Build history of the part. All positions in model axes, mm. Round coordinates to 2 decimals unless told otherwise and drop trailing zeros. Write each question's results on one line, items separated by ' | '. Start each with the question number.
```python
from build123d import *

# Parameters (mm, degrees)
SKETCH1_W            = 203.2
SKETCH1_H            = 177.8
SKETCH1_W_2          = 15.24
SKETCH1_H_2          = 17.78
BOSS_EXTRUDE1_DEPTH  = 2.54
LPATTERN2_COUNT      = 9
LPATTERN2_PITCH      = 20
LPATTERN2_COUNT_DIR2 = 10
LPATTERN2_PITCH_DIR2 = 20


with BuildPart() as part:
    # Sketch1 → Boss-Extrude1 (new body)
    with BuildSketch(Plane.XY):
        Rectangle(SKETCH1_W, SKETCH1_H)
        with Locations((-30.48, 0)):
            Rectangle(SKETCH1_W_2, SKETCH1_H_2, mode=Mode.SUBTRACT)
        with Locations((30.48, 0)):
            Rectangle(SKETCH1_W_2, SKETCH1_H_2, mode=Mode.SUBTRACT)
    extrude(amount=BOSS_EXTRUDE1_DEPTH)

    # Sketch4 → M2.5 Clearance Hole1 (revolve, cut)
    with BuildSketch(Plane(origin=(91.6, 78.994, 0), x_dir=(0, 1, 0), z_dir=(1, 0, 0))):
        Polygon((0, 0), (0, 5.623506083), (1.75, 4.572), (1.75, 0), align=None)
    m2_5_clearance_hole1 = revolve(axis=Axis((91.6, 78.994, -6.35), (0, 0, 1)), mode=Mode.SUBTRACT)

    # LPattern2: M2.5 Clearance Hole1 9 × 10, 8 skipped
    with Locations(*[(-j * LPATTERN2_PITCH_DIR2, -i * LPATTERN2_PITCH, 0) for i in range(LPATTERN2_COUNT) for j in range(LPATTERN2_COUNT_DIR2) if (i, j) not in ((0, 0), (4, 3), (4, 4), (4, 5), (4, 6), (5, 3), (5, 4), (5, 5), (5, 6))]):
        add(m2_5_clearance_hole1, mode=Mode.SUBTRACT)


solid = part.part
```
Item 1: Saw through at A-A, the plane z = 1.4. State how many separate pieces and enclosed holes the cut face has, then the cut area to 3 significant figures.
Item 2: Drill centre line: line 1 along X through (y, z) = (-6.5, 1.55). Where is it in solid material? Low to high. Write a range as [from, to].
Item 3: Drop a flat-ended pin along its axis: pin 1 (3 mm diameter, centred on x = 51.6, y = -21.006, fed in from -Z). Give the stop position or say it passes through.
Working result:
1) separate pieces: 1 | enclosed holes: 84 | area: 34,800 mm²
2) line 1: x = [-101.6, -38.1], [-22.86, 22.86], [38.1, 101.6]
3) pin 1: passes through
